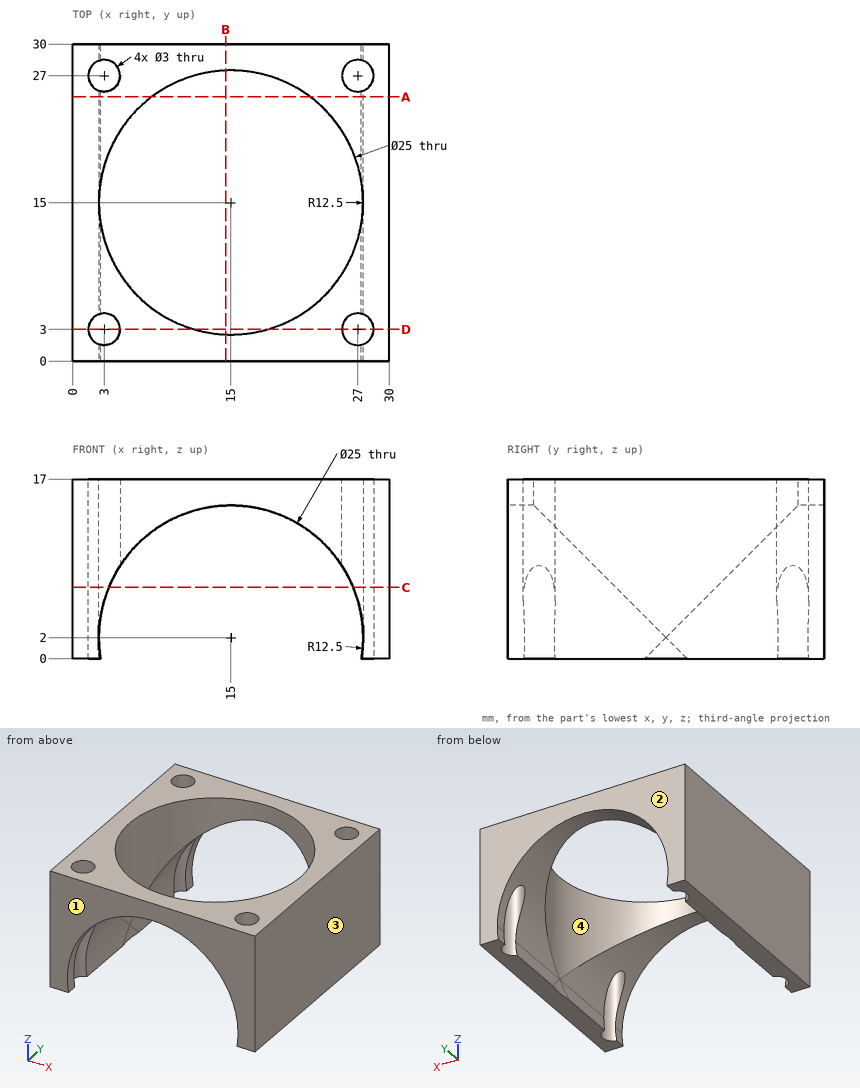
The drawing under review shows one solid part. Ordinate dimensions are in mm from its lowest x, y, z. Give positions to 0.01 mm unless a question says otherwise; leave off trailing zeros. Write each loop counter-clockwise with the first axis right and the second up, starting at its lowest first coordinate (ties: lowest second). Pieces come first, ordered by that corner, then holes.
1. Add section D-D, the plane y = 3. Write out the cut boundary in (x, z), plus the area to 3 significant figures.
2. Wall thickness on L1, parallel to X at y = 17, z = 8; L2, parallel to X at y = 22, z = 1.75; L3, parallel to Y at x = 2, z = 11.75: over which ranges is each line inside the solid? List them lowest first.
3. For P1, Ø1.8, axis at x = 27, y = 3, coming from the +Z side, flat-tipped, find the tip position at first contact; note if it passes through.
4. Add section A-A, the plane y = 25. Write out the cut boundary in (x, z).
5. Add section C-C, the plane z = 6.75. Write out the cut boundary in (x, y).
6. Add section B-B, the plane x = 14.5. Write out the cut boundary in (y, z).
7. Draft analysis for pull direction Y (two halves, no side actions). For the marked faces 1, 2, 3 and 4, state which applies: +Y half, -Y half, draft (parallel to the pull), parting line (faces both ways), or undercut.
Worked answers:
1. outline: (0, 0) - (1.5, 0) - (1.5, 17) - (0, 17) - close; (4.5, 8.78) arc R12.5 cw to (11.5, 14) - (11.5, 17) - (4.5, 17) - close; (18.5, 14) arc R12.5 cw to (25.5, 8.78) - (25.5, 17) - (18.5, 17) - close; (28.5, 0) - (30, 0) - (30, 17) - (28.5, 17) - close
1. area: 120 mm2
2. L1: x = 0 to 2.66, 27.34 to 30
2. L2: x = 0 to 2.5, 27.5 to 30
2. L3: y = 0 to 1.88, 4.12 to 25.88, 28.12 to 30
3. P1: passes through
4. outline: (0, 0) - (2.66, 0) arc R12.5 cw to (7.5, 12) - (7.5, 17) - (0, 17) - close; (22.5, 12) arc R12.5 cw to (27.34, 0) - (30, 0) - (30, 17) - (22.5, 17) - close
5. outline: (0, 0) - (3.44, 0) - (3.44, 1.57) arc R1.5 cw (long way) to (3.44, 4.43) - (3.44, 10.25) arc R12.5 cw to (3.44, 19.75) - (3.44, 25.57) arc R1.5 cw (long way) to (3.44, 28.43) - (3.44, 30) - (0, 30) - close; (26.56, 0) - (30, 0) - (30, 30) - (26.56, 30) - (26.56, 28.43) arc R1.5 cw (long way) to (26.56, 25.57) - (26.56, 19.75) arc R12.5 cw to (26.56, 10.25) - (26.56, 4.43) arc R1.5 cw (long way) to (26.56, 1.57) - close
6. outline: (0, 14.49) - (2.51, 14.49) - (2.51, 17) - (0, 17) - close; (27.49, 14.49) - (30, 14.49) - (30, 17) - (27.49, 17) - close
7. face 1: -Y half
7. face 2: +Y half
7. face 3: draft
7. face 4: undercut
